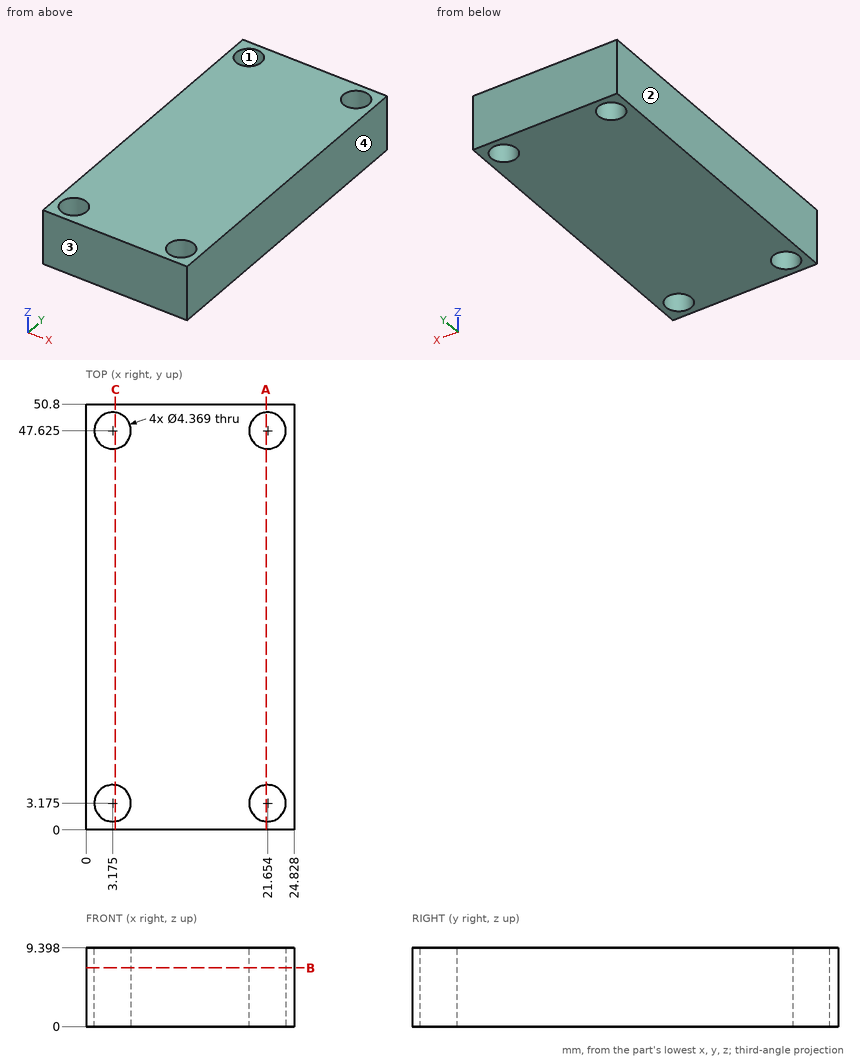
Can you work these out from the drawing? Everything is in mm from the part's minimum corner. Round coordinates to 2 decimals unless told otherwise and drop trailing zeros. Order: outer loops, then holes, each group sorted by start corner. A loop starts at its lowest first (then second) coordinate and runs counter-clockwise, first axis right, second up. Notation, with made-up numbers: M 38.5,48.25 L 62.5,48.25 A7 ccw 62.5,54.25 Z; hole C 2,-6.5 d5. An arc over 180 degrees is marked long. Answer as CSV lines item,"result".
Item 1: We'd pull the mould along X, two halves only. Please class the marked faces 1, 2, 3 and 4: +X half, -X half, draft (parallel to the pull), parting line (faces both ways), or undercut.
From the geometry:
face 1,"undercut"
face 2,"-X half"
face 3,"draft"
face 4,"+X half"
Item 2: Please list where these lines run through material, in increasing order: L1, parallel to Y at x = 21.5, z = 5.25 (1 decimal); L2, parallel to X at y = 3, z = 3.5 (1 decimal); L3, parallel to X at y = 4, z = 2.75 (1 decimal). Write a range as [from, to].
From the geometry:
L1,"[0, 1], [5.4, 45.4], [49.8, 50.8]"
L2,"[0, 1], [5.4, 19.5], [23.8, 24.8]"
L3,"[0, 1.2], [5.2, 19.6], [23.7, 24.8]"
Item 3: For pin 1 (3.5 mm diameter, centred on x = 3.17, y = 3.17, fed in from +Z) (1 decimal), with a flat end and sliding along its axis, tell me the tip position at first contact or that it passes through.
From the geometry:
pin 1,"through"
Item 4: Imagine slicing it at C-C on x = 3.5. List the corners of the cut face in (y, z) for me (1 decimal), and give its area (3 significant figures).
From the geometry:
outline,"M 0,0 L 1,0 L 1,9.4 L 0,9.4 Z; M 5.3,0 L 45.5,0 L 45.5,9.4 L 5.3,9.4 Z; M 49.8,0 L 50.8,0 L 50.8,9.4 L 49.8,9.4 Z"
area,"396 mm2"
Item 5: Imagine slicing it at B-B on z = 7. List the corners of the cut face in (x, y) for me (1 decimal), and give its area (3 significant figures).
From the geometry:
outline,"M 0,0 L 24.8,0 L 24.8,50.8 L 0,50.8 Z; hole C 3.2,3.2 d4.4; hole C 3.2,47.6 d4.4; hole C 21.7,3.2 d4.4; hole C 21.7,47.6 d4.4"
area,"1,200 mm2"
Item 6: Imagine slicing it at A-A on x = 21.5. List the corners of the cut face in (y, z) for me (1 decimal).
From the geometry:
outline,"M 0,0 L 1,0 L 1,9.4 L 0,9.4 Z; M 5.4,0 L 45.4,0 L 45.4,9.4 L 5.4,9.4 Z; M 49.8,0 L 50.8,0 L 50.8,9.4 L 49.8,9.4 Z"
